Input: part model. Units: mm. Frame: model coordinates. Face numbers are marked on the shaded views. A direction names the side the tool comes from. Coordinates: 2 decimals unless noted, no trailing zeros. Order: outer loops, then holes, each group sorted by start corner. A loop starts at its lowest first (then second) coordinate and runs counter-clockwise, first axis right, second up. Notation, with made-up numbers: M -9,26 L 4,26 A21 ccw 4,40 Z; hole C 73.25,-40 d10. An arc over 180 degrees is marked long. One line per item, written item: value.
```python
from build123d import *

# Parameters (mm, degrees)
SKETCH1_W               = 30
SKETCH1_H               = 40
BOSS_EXTRUDE1_DEPTH     = 3.175
SKETCH3_W               = 30
SKETCH3_H               = 3.175
BOSS_EXTRUDE2_DEPTH     = 10
CUT_EXTRUDE1_DEPTH      = 45.705487639
CUT_EXTRUDE1_DEPTH_BACK = 45.705487639
SKETCH4_R               = 1.5


with BuildPart() as part:
    # Sketch1 → Boss-Extrude1 (new body)
    with BuildSketch(Plane.XY):
        Rectangle(SKETCH1_W, SKETCH1_H)
    extrude(amount=BOSS_EXTRUDE1_DEPTH)

    # Sketch3 → Boss-Extrude2 (add)
    with BuildSketch(Plane.XY.offset(3.175)):
        with Locations((0, 18.4125)):
            Rectangle(SKETCH3_W, SKETCH3_H)
        with Locations((0, -18.4125)):
            Rectangle(SKETCH3_W, SKETCH3_H)
    extrude(amount=BOSS_EXTRUDE2_DEPTH)

    # Sketch4 → Cut-Extrude1 (cut, two sides: drawn at the far end of the back side and taken through both)
    with BuildSketch(Plane(origin=(0, 20, 0), x_dir=(1, 0, 0), z_dir=(0, 1, 0)).offset(-CUT_EXTRUDE1_DEPTH_BACK)):
        with Locations(Location((-8, -8, 0), (0, 0, 270))):
            Circle(SKETCH4_R)
        with Locations(Location((8, -8, 0), (0, 0, 270))):
            Circle(SKETCH4_R)
    extrude(amount=CUT_EXTRUDE1_DEPTH + CUT_EXTRUDE1_DEPTH_BACK, mode=Mode.SUBTRACT)


solid = part.part
```
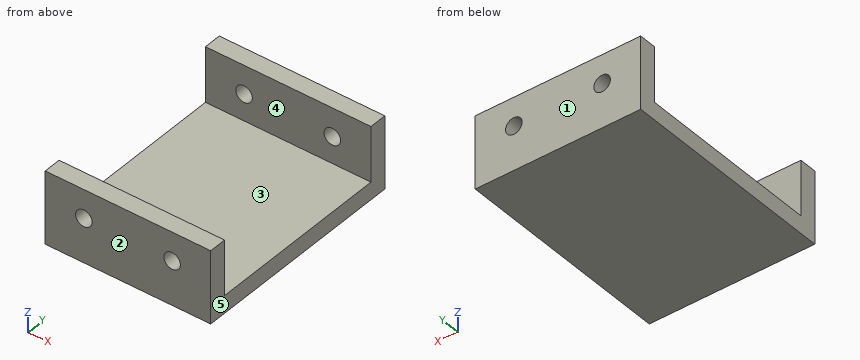
(1) Cut plane C-C on z = 5.25. Output: boundary loops of the cut face in (x, y) (3 decimals), plus the area to 4 significant figures.
Data:
outline: M -15,-20 L 15,-20 L 15,-16.825 L -15,-16.825 Z; M -15,16.825 L 15,16.825 L 15,20 L -15,20 Z
area: 190.5 mm2
(2) First-contact query: pin 1 (1 mm diameter, centred on x = -8, z = 7.5, fed in from +Y); pin 2 (1.5 mm diameter, centred on x = -1, y = 9, fed in from +Z) (3 decimals). Flat tips, straight axial feed; report the tip coordinate or a pass-through.
Data:
pin 1: passes through
pin 2: stops at z = 3.175
(3) Cut plane B-B on z = 8. Output: boundary loops of the cut face in (x, y) (3 decimals), plus the area to 3 significant figures.
Data:
outline: M -15,-20 L -9.5,-20 L -9.5,-16.825 L -15,-16.825 Z; M -15,16.825 L -9.5,16.825 L -9.5,20 L -15,20 Z; M -6.5,-20 L 6.5,-20 L 6.5,-16.825 L -6.5,-16.825 Z; M -6.5,16.825 L 6.5,16.825 L 6.5,20 L -6.5,20 Z; M 9.5,-20 L 15,-20 L 15,-16.825 L 9.5,-16.825 Z; M 9.5,16.825 L 15,16.825 L 15,20 L 9.5,20 Z
area: 152 mm2
(4) Ray query, line 1 (X direction, y = 17.65, z = 8); line 2 (Y direction, x = 10.5, z = 6.75) (3 decimals); line 3 (Z direction, x = -8, y = -19.2) (3 decimals). Return the intervals inside material, ascending. Write a range as from..to.
Data:
line 1: x = -15..-9.5, -6.5..6.5, 9.5..15
line 2: y = -20..-16.825, 16.825..20
line 3: z = 0..6.5, 9.5..13.175
(5) Cut plane D-D on x = 3.5. Output: boundary loops of the cut face in (y, z) (3 decimals).
Data:
outline: M -20,0 L 20,0 L 20,13.175 L 16.825,13.175 L 16.825,3.175 L -16.825,3.175 L -16.825,13.175 L -20,13.175 Z
(6) Cut plane A-A on x = 8. Output: boundary loops of the cut face in (y, z) (3 decimals), plus the area to 3 significant figures.
Data:
outline: M -20,0 L 20,0 L 20,6.5 L 16.825,6.5 L 16.825,3.175 L -16.825,3.175 L -16.825,6.5 L -20,6.5 Z; M -20,9.5 L -16.825,9.5 L -16.825,13.175 L -20,13.175 Z; M 16.825,9.5 L 20,9.5 L 20,13.175 L 16.825,13.175 Z
area: 171 mm2
(7) Draft query along Y for the marked faces 1, 2 and 3. Return one class per face: released by +Y, released by -Y, zero draft, split by the parting line, or undercut.
Data:
face 1: released by +Y
face 2: released by -Y
face 3: undercut
(8) Access query for the marked faces 4 and 5. Directions: +Z, -Z, +X, -X, +Y, -Y. A direction counts if a zero-diameter tool reaches every point of the face in a straight line with its end or side. Return the directions, or none.
Data:
face 4: +Z, +X, -X
face 5: +Z, -Z, +X, +Y, -Y
